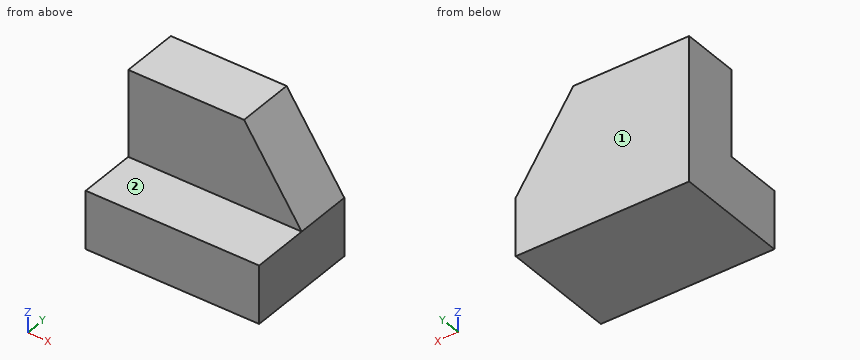
from build123d import *

# Parameters (mm, degrees)
F2_DEPTH = 25.4
F0_W     = 38.1
F0_H     = 31.75
F3_DEPTH = 25.4
F4_W     = 38.1
F4_H     = 18.9845859185
F5_DEPTH = 12.7
F7_DEPTH = 12.701


with BuildPart() as f2:
    # F1 (on Front) → F2 (new body)
    with BuildSketch(Plane.XZ):
        Polygon((33.8248718529, 28.3878277987), (0, 28.3878277987), (0, 0), (34.039542079, 0), align=None)
    extrude(amount=F2_DEPTH)

    # F0 (on Front) → F3 (join)
    with BuildSketch(Plane.XZ):
        with Locations((19.05, 15.875)):
            Rectangle(F0_W, F0_H)
    extrude(amount=F3_DEPTH)

    # F4 (on face) → F5 (cut)
    with BuildSketch(Plane.XZ.offset(25.4)):
        with Locations((19.05, 22.2577070408)):
            Rectangle(F4_W, F4_H)
    extrude(amount=-F5_DEPTH, mode=Mode.SUBTRACT)

    # F6 (on face) → F7 (cut, through all)
    with BuildSketch(Plane.XZ.offset(12.7)):
        Polygon((38.1, 31.75), (25.4303161055, 31.75), (38.1, 12.7654140815), align=None)
    extrude(amount=-F7_DEPTH, mode=Mode.SUBTRACT)


solid = f2.part
Verification items for the finished model (mm, model axes). Face numbers are marked on the shaded views. A direction names the side the tool comes from. Coordinates: 2 decimals unless noted, no trailing zeros. Loops run counter-clockwise (first coordinate to the right, second up) from the corner with the lowest first, then second, coordinate; pieces in that order, holes last. Notation, with made-up numbers: M -22,-30.75 L -10,-30.75 A25 ccw -10,-4.75 Z; hole C -24.75,24.5 d9. An arc over 180 degrees is marked long. One line per item, written item: value.
1. Section check B-B on x = 11.5. Record the cut outline in (y, z), plus the area to 3 significant figures.
Answers follow:
outline: M -25.4,0 L 0,0 L 0,31.75 L -12.7,31.75 L -12.7,12.77 L -25.4,12.77 Z
area: 565 mm^2
2. Gauge pin test, flat ends, axial feed: P1, Ø6, axis at x = 18, y = -16.5, coming from the +Z side; P2, Ø9.5, axis at x = 15.5, z = 24, coming from the -Y side. Record the tip position at first contact, or that the pin passes through.
Answers follow:
P1: z = 12.77
P2: y = -12.7
3. Section check D-D on y = -20. Record the cut outline in (x, z).
Answers follow:
outline: M 0,0 L 38.1,0 L 38.1,12.77 L 0,12.77 Z
4. Set-up check for the marked faces 1 and 2: record each of +Z, -Z, +X, -X, +Y, -Y from which the full face is reachable in a straight line by a thin tool's end or side.
Answers follow:
face 1: +Z, -Z, +X, -X, +Y
face 2: +Z, +X, -X, -Y
5. Material ranges on line 1 along Y through (x, z) = (18, 29.5); line 2 along Z through (x, y) = (35.5, -24); line 3 along X through (y, z) = (-6, 13), recorded low to high. Write a range as from..to.
Answers follow:
line 1: -12.7..0
line 2: 0..12.77
line 3: 0..37.94
6. Section check C-C on z = 26. Record the cut outline in (x, y).
Answers follow:
outline: M 0,-12.7 L 29.27,-12.7 L 29.27,0 L 0,0 Z
7. Section check A-A on y = -4. Record the cut outline in (x, z), plus the area to 3 significant figures.
Answers follow:
outline: M 0,0 L 38.1,0 L 38.1,12.77 L 25.43,31.75 L 0,31.75 Z
area: 1,090 mm^2
